```python
from build123d import *

# Parameters (mm, degrees)
ESBO_O1_W                = 116
ESBO_O1_H                = 216.23
ESBO_O1_R                = 1.75
ESBO_O1_W_2              = 50
ESBO_O1_H_2              = 50
RESSALTO_EXTRUS_O2_DEPTH = 8
ESBO_O2_R                = 1.75
CORTE_EXTRUS_O1_DEPTH    = 100
PADR_O_LINEAR1_COUNT     = 8
PADR_O_LINEAR1_PITCH     = 12.714285714
ESBO_O3_R                = 1.75
CORTE_EXTRUS_O2_DEPTH    = 100
PADR_O_LINEAR2_COUNT     = 8
PADR_O_LINEAR2_PITCH     = 12.714285714


with BuildPart() as part:
    # Esboço1 → Ressalto-extrusão2 (new body)
    with BuildSketch(Plane.XY):
        with Locations((18, -68.115)):
            Rectangle(ESBO_O1_W, ESBO_O1_H)
        with Locations((-17, 32)):
            Circle(ESBO_O1_R, mode=Mode.SUBTRACT)
        with Locations((17, 32)):
            Circle(ESBO_O1_R, mode=Mode.SUBTRACT)
        with Locations((-17, -32)):
            Circle(ESBO_O1_R, mode=Mode.SUBTRACT)
        with Locations((17, -32)):
            Circle(ESBO_O1_R, mode=Mode.SUBTRACT)
        Rectangle(ESBO_O1_W_2, ESBO_O1_H_2, mode=Mode.SUBTRACT)
    extrude(amount=RESSALTO_EXTRUS_O2_DEPTH)

    # Esboço2 → Corte-extrusão1 (cut)
    with BuildSketch(Plane(origin=(0, 0, 0), x_dir=(-1, 0, 0), z_dir=(0, 0, -1))):
        with Locations((-66.5, -166.73)):
            Circle(ESBO_O2_R)
    corte_extrus_o1 = extrude(amount=-CORTE_EXTRUS_O1_DEPTH, mode=Mode.SUBTRACT)

    # Padrão linear1: Corte-extrusão1 ×8
    with Locations(*[(-i * PADR_O_LINEAR1_PITCH, 0, 0) for i in range(1, PADR_O_LINEAR1_COUNT)]):
        add(corte_extrus_o1, mode=Mode.SUBTRACT)

    # Esboço3 → Corte-extrusão2 (cut)
    with BuildSketch(Plane(origin=(0, 0, 0), x_dir=(-1, 0, 0), z_dir=(0, 0, -1))):
        with Locations((22.5, -55.5)):
            Circle(ESBO_O3_R)
    corte_extrus_o2 = extrude(amount=-CORTE_EXTRUS_O2_DEPTH, mode=Mode.SUBTRACT)

    # Padrão linear2: Corte-extrusão2 ×8
    with Locations(*[(0, -i * PADR_O_LINEAR2_PITCH, 0) for i in range(1, PADR_O_LINEAR2_COUNT)]):
        add(corte_extrus_o2, mode=Mode.SUBTRACT)


solid = part.part
```
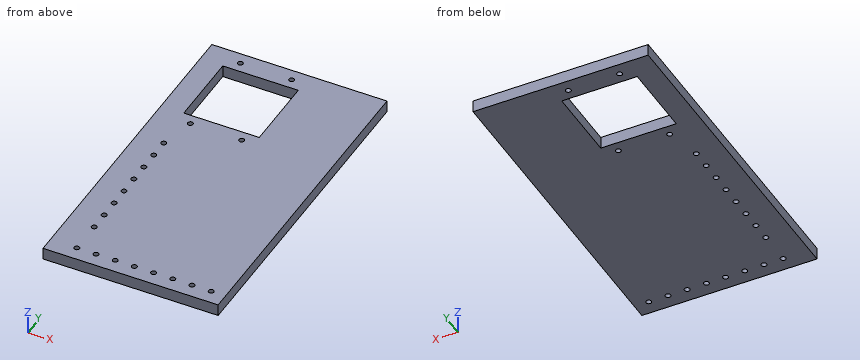
Geometry check sheet. Reference: the model listing, model coordinates, mm. Coordinates: 2 decimals unless noted, no trailing zeros. Write each loop counter-clockwise with the first axis right and the second up, starting at its lowest first coordinate (ties: lowest second). Pieces come first, ordered by that corner, then holes. Notation, with made-up numbers: (-37.75, -24.75) -> (16.25, -24.75) arc R16 ccw to (16.25, -14.75) -> close; hole circle Ø3 at (10, 35.5). An arc over 180 degrees is marked (long way). Use CSV: the item, a comma, the result in double quotes. Start each with the question number.
Item 1: Depth check by flat-ended pin: pin 1 Ø3 at (x, y) = (-22.5, -106.36) entering from -Z. Enter the tip coordinate at first touch or a pass-through.
Item 2: Cross-section at B-B, the plane z = 6. State how many separate pieces and enclosed holes the cut face has, plus the area to 3 significant figures.
Item 3: Thickness scan on line 1 (X direction, y = -3, z = 2); line 2 (Y direction, x = -4, z = 5); line 3 (Y direction, x = 42.5, z = 0.75). Record the ranges inside material, lowest first.
Item 4: Cross-section at A-A, the plane y = -1. Record the cut outline in (x, z), plus the area to 3 significant figures.
Answers:
1,pin 1,"through"
2,separate pieces,"1"
2,enclosed holes,"21"
2,area,"22,400 mm^2"
3,line 1,"-40 to -25, 25 to 76"
3,line 2,"-176.23 to -25, 25 to 40"
3,line 3,"-176.23 to -167.74, -165.72 to 40"
4,outline,"(-40, 0) -> (-25, 0) -> (-25, 8) -> (-40, 8) -> close; (25, 0) -> (76, 0) -> (76, 8) -> (25, 8) -> close"
4,area,"528 mm^2"
